Here's how the part is built. I have some questions about the finished solid (model axes, mm). Face numbers are marked on the shaded views. Round coordinates to 2 decimals unless told otherwise and drop trailing zeros. One line per item, written item: value. Start each with the question number.
Item 1: If I drill on line 1 (Z direction, x = -11, y = -11.5); line 2 (X direction, y = -1.5, z = 3); line 3 (Y direction, x = -2.5, z = -19), over which ranges is the centre line in solid material (lowest first)?
Item 2: For P1, Ø4, axis at y = 1, z = 2, coming from the -X side; P2, Ø1.5, axis at y = 3.5, z = 2, coming from the +X side; P3, Ø2, axis at x = 7, z = -9, coming from the -Y side, each with a flat end and sliding along its axis, tell me the tip position at first contact or that it passes through.
Item 3: Thinking about a two-plate mould opening in Y: for the marked faces 1 and 2, which applies, released by +Y, released by -Y, zero draft, split by the parting line, or undercut?
```python
from build123d import *

# Parameters (mm, degrees)
F4_W     = 40
F4_H     = 40
F5_W     = 36
F5_H     = 36
F0_W     = 32
F0_H     = 32
F7_DEPTH = 25
F8_R     = 4
F9_R     = 1


with BuildPart() as f6:
    # F4 (on plane+point) → F6 section 0
    with BuildSketch(Plane.XY.offset(-29)):
        Rectangle(F4_W, F4_H)
    # F5 (on offset) → F6 section 1
    with BuildSketch(Plane.XY.offset(5)):
        Rectangle(F5_W, F5_H)
    loft()

    # F0 (on Top) → F7 (cut)
    with BuildSketch(Plane.XY):
        Rectangle(F0_W, F0_H)
    extrude(amount=F7_DEPTH, mode=Mode.SUBTRACT)

    # F8
    f8_edges = [f6.edges().sort_by_distance(p)[0] for p in [
        (19, -19, -12),
        (19, 19, -12),
        (-19, -19, -12),
        (-19, 19, -12),
    ]]
    fillet(f8_edges, radius=F8_R)

    # F9
    f9_edges = [f6.edges().sort_by_distance(p)[0] for p in [
        (-16, 16, 2.5),
        (16, 16, 2.5),
        (16, -16, 2.5),
        (-16, -16, 2.5),
    ]]
    fillet(f9_edges, radius=F9_R)


solid = f6.part
```
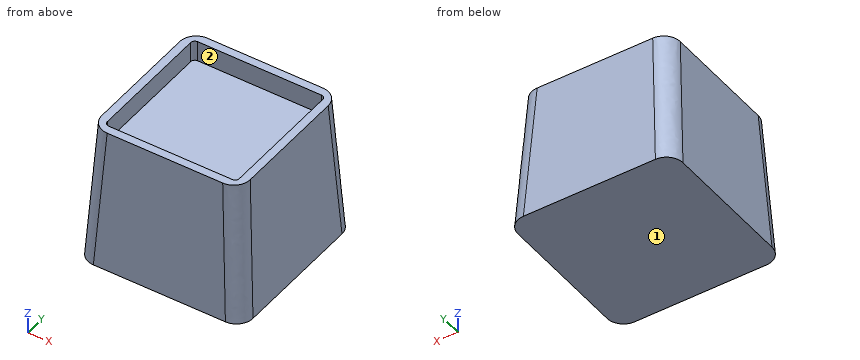
Values follow:
1. line 1: z = -29 to 0
1. line 2: x = -18.12 to -16, 16 to 18.12
1. line 3: y = -19.41 to 19.41
2. P1: stops at x = -18.29
2. P2: stops at x = 18.22
2. P3: stops at y = -18.88
3. face 1: zero draft
3. face 2: undercut
